Build history of the part. All positions in model axes, mm. A direction names the side the tool comes from. Coordinates: 2 decimals unless noted, no trailing zeros. Order: outer loops, then holes, each group sorted by start corner. A loop starts at its lowest first (then second) coordinate and runs counter-clockwise, first axis right, second up. Notation, with made-up numbers: (62.25, -30.5) - (99.25, -30.5) arc R21 ccw to (99.25, -12.5) - close; hole circle Ø6 at (62.5, 54.5). An arc over 180 degrees is marked (long way). One line per item, written item: value.
Autodesk Inventor part; units mm, degrees
ref_plane "YZ Plane" through (0, 0, 0) normal (1, 0, 0) x (0, 1, 0)
ref_plane "XZ Plane" through (0, 0, 0) normal (0, 1, 0) x (-1, 0, 0)
ref_plane "XY Plane" through (0, 0, 0) normal (0, 0, 1) x (1, 0, 0)
sketch "Sketch1" plane through (0, 0, 0) normal (1, 0, 0) x (0, 1, 0)
  line L0 (0, 0) -> (11.5, 0)
  line L1 (11.5, 0) -> (11.5, 31)
  line L2 (11.5, 31) -> (0, 31)
  line L3 (0, 20) -> (-11.6, 20)
  line L4 (-11.6, 20) -> (-11.6, 10)
  line L5 (-11.6, 10) -> (0, 10)
  line L6 (0, 31) -> (0, 20)
  line L7 (0, 10) -> (0, 0)
  line L8 (7, 31) -> (7, 0) construction
  circle A0 centre (7, 26) radius 1.8
  circle A1 centre (7, 5.5) radius 1.8
  line L9 (-11.6, 15) -> (4, 15) construction
  circle A2 centre (4, 15) radius 1.5
  line L10 (-5.6, 12.85) -> (-9.6, 12.85)
  line L11 (-9.6, 12.85) -> (-9.6, 17.15)
  line L12 (-9.6, 17.15) -> (-5.6, 17.15)
  line L13 (-5.6, 17.15) -> (-5.6, 12.85)
  line L14 (-5.6, 12.85) -> (-9.6, 17.15) construction
  line L15 (-9.6, 12.85) -> (-5.6, 17.15) construction
  point P0 (-7.6, 15)
  dimension "d0" = 10
  dimension "d4" = 11.5
  dimension "d7" = 20.5
  dimension "d8" = 3.6
  dimension "d10" = 7
  dimension "d11" = 3
  dimension "d12" = 4
  dimension "d13" = 9.5
  dimension "d14" = 16
  dimension "d15" = 15
  dimension "d16" = 5.6
  dimension "d17" = 4
  dimension "d18" = 4.3
  dimension "d19" = 2
extrude "Extrusion1" add sketch "Sketch1" along normal blind 4.3
properties part number "TrayPanelI"
1. Flat gauge pins, fed straight in: P1, Ø1.3, axis at x = 1.5, z = 4.5, coming from the -Y side; P2, Ø1, axis at x = 1.5, y = -6, coming from the -Z side; P3, Ø2, axis at x = 1.5, y = -8.5, coming from the +Z side. Where does each tip first touch, or does it go through?
Values found:
P1: stops at y = 0
P2: stops at z = 10
P3: stops at z = 20
2. Two-plate mould, pull along Z, no slides. Class faces 1 (the face through (2, -6, 10)), 2 (the face through (2, -9.6, 15)), 3 (the face through (2, -6, 20)), 4 (the face through (2, 0, 26)): pulls with the +Z half, pulls with the -Z half, needs draft (parallel to the pull), parting line crosses it, or undercut.
Values found:
face 1: pulls with the -Z half
face 2: undercut
face 3: pulls with the +Z half
face 4: needs draft
3. Band-saw the part on D-D, the plane y = 4. Give the cut face in (x, z).
Values found:
outline: (0, 0) - (4.3, 0) - (4.3, 13.5) - (0, 13.5) - close; (0, 16.5) - (4.3, 16.5) - (4.3, 31) - (0, 31) - close
4. 3-axis set-ups, long thin cutter, end or side, ignore diameter. For faces 5 (the face through (2, -8, 12.85)), 6 (the face through (4.3, 2, 16)), 7 (the face through (2, 0, 5)): which of +Z, -Z, +X, -X, +Y, -Y reach the whole face in a straight line?
Values found:
face 5: +X, -X
face 6: +Z, -Z, +X, +Y, -Y
face 7: -Z, +X, -X, -Y
5. Band-saw the part on A-A, the plane z = 15. Give the cut face in (x, y).
Values found:
outline: (0, -11.6) - (4.3, -11.6) - (4.3, -9.6) - (0, -9.6) - close; (0, -5.6) - (4.3, -5.6) - (4.3, 2.5) - (0, 2.5) - close; (0, 5.5) - (4.3, 5.5) - (4.3, 11.5) - (0, 11.5) - close
6. Band-saw the part on B-B, the plane y = 7. Give the cut face in (x, z).
Values found:
outline: (0, 0) - (4.3, 0) - (4.3, 3.7) - (0, 3.7) - close; (0, 7.3) - (4.3, 7.3) - (4.3, 24.2) - (0, 24.2) - close; (0, 27.8) - (4.3, 27.8) - (4.3, 31) - (0, 31) - close
7. Probe line 1 along Z through (x, y) = (1.35, 7); line 2 along Z through (x, y) = (2.55, 4); line 3 along Z through (x, y) = (2.5, -6). List the from-to ranges inside material, lowest first.
Values found:
line 1: z = 0 to 3.7, 7.3 to 24.2, 27.8 to 31
line 2: z = 0 to 13.5, 16.5 to 31
line 3: z = 10 to 12.85, 17.15 to 20
8. Band-saw the part on C-C, the plane z = 5.5. Give the cut face in (x, y).
Values found:
outline: (0, 0) - (4.3, 0) - (4.3, 5.2) - (0, 5.2) - close; (0, 8.8) - (4.3, 8.8) - (4.3, 11.5) - (0, 11.5) - close
